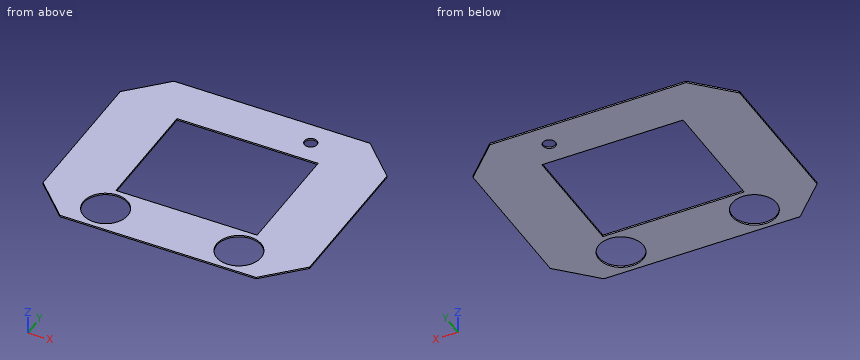
Autodesk Inventor part; units mm, degrees
ref_plane "YZ Plane" through (0, 0, 0) normal (1, 0, 0) x (0, 1, 0)
ref_plane "XZ Plane" through (0, 0, 0) normal (0, 1, 0) x (-1, 0, 0)
ref_plane "XY Plane" through (0, 0, 0) normal (0, 0, 1) x (1, 0, 0)
sketch "Эскиз1" plane through (0, 0, 0) normal (0, 0, 1) x (1, 0, 0)
  line L0 (0, 0) -> (250, 0)
  line L1 (250, 0) -> (250, 280)
  line L2 (250, 280) -> (0, 280)
  line L3 (0, 280) -> (0, 0)
  line L4 (250, 280) -> (295, 235)
  line L5 (295, 235) -> (295, 45)
  line L6 (295, 45) -> (250, 0)
  line L7 (0, 0) -> (-45, 45)
  line L8 (-45, 45) -> (-45, 235)
  line L9 (-45, 235) -> (0, 280)
  line L10 (35, 220) -> (215, 220)
  line L11 (215, 220) -> (215, 70)
  line L12 (215, 70) -> (35, 70)
  line L13 (35, 70) -> (35, 220)
  circle A0 centre (40, 35) radius 28.3
  circle A1 centre (210, 35) radius 28.3
  line L14 (125, 280) -> (125, 0) construction
  line L15 (40, 35) -> (210, 35) construction
  circle A2 centre (190, 250) radius 8.05
  point P0 (125, 220)
  point P1 (125, 35)
  dimension "d0" = 45
  dimension "d1" = 280
  dimension "d2" = 250
  dimension "d4" = 45
  dimension "d5" = 70
  dimension "d6" = 150
  dimension "d7" = 180
  dimension "d8" = 56.6
  dimension "d9" = 35
  dimension "d11" = 170
  dimension "d14" = 16.1
  dimension "d15" = 30
  dimension "d16" = 60
extrude "Выдавливание1" add sketch "Эскиз1" along normal blind 2
properties part number "face"
Model file for the job. Use its own axes, mm. Coordinates: 2 decimals unless noted, no trailing zeros. Order: outer loops, then holes, each group sorted by start corner. A loop starts at its lowest first (then second) coordinate and runs counter-clockwise, first axis right, second up. Notation, with made-up numbers: M -7,-9.75 L 47,-9.75 A34 ccw 47,22.25 Z; hole C 21.25,16 d5. An arc over 180 degrees is marked long. Answer as CSV lines item,"result".
(1) Band-saw the part on C-C, the plane y = 35. List the corners of the cut face in (x, z), then the cut area to 3 significant figures.
Geometry says:
outline,"M -35,0 L 11.7,0 L 11.7,2 L -35,2 Z; M 68.3,0 L 181.7,0 L 181.7,2 L 68.3,2 Z; M 238.3,0 L 285,0 L 285,2 L 238.3,2 Z"
area,"414 mm2"
(2) Band-saw the part on A-A, the plane y = 250. List the corners of the cut face in (x, z), then the cut area to 3 significant figures.
Geometry says:
outline,"M -30,0 L 181.95,0 L 181.95,2 L -30,2 Z; M 198.05,0 L 280,0 L 280,2 L 198.05,2 Z"
area,"588 mm2"
(3) Wall check: line 1 along Y through (x, z) = (40, 0.4); line 2 along X through (y, z) = (211, 1.7); line 3 along X through (y, z) = (32.5, 1.75). Give the ranges that are in metal, low to high.
Geometry says:
line 1,"y = 0 to 6.7, 63.3 to 70, 220 to 280"
line 2,"x = -45 to 35, 215 to 295"
line 3,"x = -32.5 to 11.81, 68.19 to 181.81, 238.19 to 282.5"
(4) Band-saw the part on B-B, the plane x = 40. List the corners of the cut face in (y, z).
Geometry says:
outline,"M 0,0 L 6.7,0 L 6.7,2 L 0,2 Z; M 63.3,0 L 70,0 L 70,2 L 63.3,2 Z; M 220,0 L 280,0 L 280,2 L 220,2 Z"
(5) Band-saw the part on D-D, the plane x = 141. List the corners of the cut face in (y, z), then the cut area to 3 significant figures.
Geometry says:
outline,"M 0,0 L 70,0 L 70,2 L 0,2 Z; M 220,0 L 280,0 L 280,2 L 220,2 Z"
area,"260 mm2"
